Part model, mm, in its own coordinate system. A direction names the side the tool comes from. Coordinates: 2 decimals unless noted, no trailing zeros. Write each loop counter-clockwise with the first axis right and the second up, starting at its lowest first coordinate (ties: lowest second). Pieces come first, ordered by that corner, then holes. Notation, with made-up numbers: (11.25, 50) - (22.25, 50) arc R28 ccw to (22.25, 78) - close; hole circle Ø2 at (14, 16). An arc over 180 degrees is marked (long way). Write each question's results on one line, items separated by ' | '.
from build123d import *

# Parameters (mm, degrees)
SKETCH1_W                  = 260
SKETCH1_H                  = 200
EXTRUDE1_DEPTH             = 10
SKETCH2_R                  = 79.5
EXTRUDE2_DEPTH             = 10
M4_CLEARANCE_HOLE2_DEPTH   = 10
EXTRUDE3_DEPTH             = 10
SKETCH6_W                  = 30
SKETCH6_H                  = 77.5
EXTRUDE4_DEPTH             = 10
FILLET1_R                  = 8
M4_CLEARANCE_HOLE3_D       = 4.5
M4_CLEARANCE_HOLE3_DEPTH   = 20
EXTRUDE5_DEPTH             = 10
F_12_0_12_DIAMETER_HOLE1_D = 12
CHAMFER1_SIZE              = 30
CHAMFER2_SIZE              = 1
CHAMFER3_SIZE              = 60
SKETCH16_W                 = 146
SKETCH16_H                 = 3
EXTRUDE6_DEPTH             = 10
FILLET4_R                  = 10
EXTRUDE7_DEPTH             = 10
SKETCH18_W                 = 20
SKETCH18_H                 = 10
EXTRUDE8_DEPTH             = 10
EXTRUDE9_DEPTH             = 10


# Read off the part's stored shape, not the designer's step: M4 Clearance Hole2
with BuildPart() as part:
    # Sketch1 → Extrude1 (new body)
    with BuildSketch(Plane(origin=(0, 0, 0), x_dir=(1, 0, 0), z_dir=(0, 1, 0))):
        Rectangle(SKETCH1_W, SKETCH1_H)
    extrude(amount=EXTRUDE1_DEPTH)

    # Sketch2 → Extrude2 (cut)
    with BuildSketch(Plane(origin=(0, 10, 0), x_dir=(1, 0, 0), z_dir=(0, 1, 0))):
        with Locations(Location((0, 0, 0), (0, 0, 270))):
            Circle(SKETCH2_R)
    extrude(amount=-EXTRUDE2_DEPTH, mode=Mode.SUBTRACT)

    # M4 Clearance Hole2 outline → M4 Clearance Hole2 (cut)
    with BuildSketch(Plane(origin=(0, 0, 0), x_dir=(1, 0, 0), z_dir=(0, 1, 0))):
        with BuildLine():
            ThreePointArc((-82.75, 48.75), (-85, 51), (-87.25, 48.75))
            Line((-87.25, 48.75), (-87.25, 41.25))
            ThreePointArc((-87.25, 41.25), (-85, 39), (-82.75, 41.25))
            Line((-82.75, 41.25), (-82.75, 48.75))
        make_face()
        with BuildLine():
            ThreePointArc((87.25, 48.75), (85, 51), (82.75, 48.75))
            Line((82.75, 48.75), (82.75, 41.25))
            ThreePointArc((82.75, 41.25), (85, 39), (87.25, 41.25))
            Line((87.25, 41.25), (87.25, 48.75))
        make_face()
    extrude(amount=M4_CLEARANCE_HOLE2_DEPTH, mode=Mode.SUBTRACT)

    # Sketch5 → Extrude3 (cut)
    with BuildSketch(Plane.XZ):
        with BuildLine():
            Line((-130, 2.5), (105, 2.5))
            ThreePointArc((105, 2.5), (107.5, 0), (105, -2.5))
            Line((105, -2.5), (-130, -2.5))
            Line((-130, -2.5), (-130, 2.5))
        make_face()
    extrude(amount=-EXTRUDE3_DEPTH, mode=Mode.SUBTRACT)

    # Sketch6 → Extrude4 (cut)
    with BuildSketch(Plane.XZ):
        with Locations((-115, 61.25)):
            Rectangle(SKETCH6_W, SKETCH6_H)
    extrude(amount=-EXTRUDE4_DEPTH, mode=Mode.SUBTRACT)

    # Fillet1
    fillet1_edges = [part.edges().sort_by_distance(p)[0] for p in [
        (-100, 5, 22.5),
    ]]
    fillet(fillet1_edges, radius=FILLET1_R)

    # M4 Clearance Hole3
    with Locations(Plane.XY.offset(22.5)):
        with Locations((-123, 5)):
            Hole(M4_CLEARANCE_HOLE3_D / 2, depth=M4_CLEARANCE_HOLE3_DEPTH)

    # Sketch11 → Extrude5 (cut)
    with BuildSketch(Plane.XZ):
        Polygon((-125.25, -2.5), (-125.25, -9.5), (-126.625, -9.5), (-126.625, -13.2), (-125.25, -13.2), (-125.25, -18.5), (-120.75, -18.5), (-120.75, -13.2), (-119.375, -13.2), (-119.375, -9.5), (-120.75, -9.5), (-120.75, -2.5), align=None)
    extrude(amount=-EXTRUDE5_DEPTH, mode=Mode.SUBTRACT)

    # Ø12.0 (12) Diameter Hole1 (through all)
    with Locations(Plane(origin=(-130, 20, 100), x_dir=(1, 0, 0), z_dir=(0, 1, 0))):
        with Locations((65, 165), (195, 165), (195, 35), (65, 35)):
            Hole(F_12_0_12_DIAMETER_HOLE1_D / 2)

    # Chamfer1
    chamfer1_edges = [part.edges().sort_by_distance(p)[0] for p in [
        (-100, 5, 100),
    ]]
    chamfer(chamfer1_edges, length=CHAMFER1_SIZE)

    # Chamfer2
    chamfer2_edges = [part.edges().sort_by_distance(p)[0] for p in [
        (-130, 5, 2.5),
        (-130, 5, -2.5),
        (-130, 5, 22.5),
    ]]
    chamfer(chamfer2_edges, length=CHAMFER2_SIZE)

    # Chamfer3
    chamfer3_edges = [part.edges().sort_by_distance(p)[0] for p in [
        (130, 5, 100),
    ]]
    chamfer(chamfer3_edges, length=CHAMFER3_SIZE)

    # Sketch16 → Extrude6 (cut)
    with BuildSketch(Plane(origin=(0, 10, 0), x_dir=(1, 0, 0), z_dir=(0, 1, 0))):
        with Locations((0, -98.5)):
            Rectangle(SKETCH16_W, SKETCH16_H)
    extrude(amount=-EXTRUDE6_DEPTH, mode=Mode.SUBTRACT)

    # Fillet4
    fillet4_edges = [part.edges().sort_by_distance(p)[0] for p in [
        (-100, 5, 70),
        (130, 5, 40),
        (-73, 5, 97),
        (73, 5, 97),
    ]]
    fillet(fillet4_edges, radius=FILLET4_R)

    # Sketch17 → Extrude7 (cut)
    with BuildSketch(Plane(origin=(0, 10, 0), x_dir=(1, 0, 0), z_dir=(0, 1, 0))):
        Polygon((-122.5, -2.5), (-123.5, -2.5), (-123, -3.5), align=None)
    extrude7 = extrude(amount=-EXTRUDE7_DEPTH, mode=Mode.SUBTRACT)

    # Mirror1: Extrude7 across plane
    add(extrude7.mirror(Plane(origin=(0, 0, 12.5), x_dir=(1, 0, 0), z_dir=(0, 0, -1))), mode=Mode.SUBTRACT)

    # Sketch18 → Extrude8 (add)
    with BuildSketch(Plane(origin=(0, 10, 0), x_dir=(1, 0, 0), z_dir=(0, 1, 0))):
        with Locations((0, 105)):
            Rectangle(SKETCH18_W, SKETCH18_H)
    extrude(amount=-EXTRUDE8_DEPTH)

    # Sketch19 → Extrude9 (cut)
    with BuildSketch(Plane(origin=(0, 10, 0), x_dir=(1, 0, 0), z_dir=(0, 1, 0))):
        with BuildLine():
            Line((-11.5, 100), (-10, 100))
            Line((-10, 100), (-10, 101.5))
            ThreePointArc((-10, 101.5), (-8.939339828, 98.939339828), (-11.5, 100))
        make_face()
        with BuildLine():
            Line((10, 101.5), (10, 100))
            Line((10, 100), (11.5, 100))
            ThreePointArc((11.5, 100), (8.939339828, 98.939339828), (10, 101.5))
        make_face()
    extrude(amount=-EXTRUDE9_DEPTH, mode=Mode.SUBTRACT)


solid = part.part
(1) Saw through at B-B on z = 11.5. Write the cut outline in (x, y), then the cut area to 3 significant figures.
Return value:
outline: (-130, 0) - (-78.66, 0) - (-78.66, 10) - (-130, 10) - close; (78.66, 0) - (130, 0) - (130, 10) - (78.66, 10) - close; hole circle Ø4.5 at (-123, 5) | area: 1,010 mm^2
(2) Wall check: line 1 (X direction, y = 2.25, z = -65); line 2 (Y direction, x = -123, z = 13); line 3 (X direction, y = 6, z = 65). Give the ranges that are in metal, low to high. Write a range as from..to.
Return value:
line 1: x = -130..-71, -59..-45.77, 45.77..59, 71..130 | line 2: y = 0..2.75, 7.25..10 | line 3: x = -100..-71, -59..-45.77, 45.77..59, 71..105
(3) 3-axis set-ups, long thin cutter, end or side, ignore diameter. For faces 4 (the flat face through (-126, 5, 22.5)), 5 (the flat face through (92, 5, -2.5)), 6 (the flat face through (-10, 5, -106)): which of +Z, -Z, +X, -X, +Y, -Y reach the whole face in a straight line?
Return value:
face 4: +Z, -X, +Y, -Y | face 5: -X, +Y, -Y | face 6: -Z, -X, +Y, -Y
(4) Two-plate mould, pull along Z, no slides. Class faces 1 (the cylindrical face through (129.26, 5.07, 39.63)), 2 (the flat face through (10, 5, -106)), 3 (the flat face through (-87.25, 5, -45)): released by +Z, released by -Z, zero draft, split by the parting line, or undercut.
Return value:
face 1: released by +Z | face 2: zero draft | face 3: undercut
(5) Saw through at A-A on x = 0. Write the cut outline in (y, z).
Return value:
outline: (0, -110) - (10, -110) - (10, -79.5) - (0, -79.5) - close; (0, 79.5) - (10, 79.5) - (10, 97) - (0, 97) - close
(6) Flat gauge pins, fed straight in: P1, Ø4, axis at y = 5, z = -107, coming from the +X side; P2, Ø1.1, axis at x = -120, y = 7, coming from the -Z side; P3, Ø2, axis at x = -122, y = 6, coming from the +Z side. Where does each tip first touch, or does it go through?
Return value:
P1: stops at x = 10 | P2: stops at z = -100 | P3: stops at z = 22.5
(7) Saw through at D-D on x = -48.5. Write the cut outline in (y, z).
Return value:
outline: (0, -100) - (10, -100) - (10, -62.99) - (0, -62.99) - close; (0, 62.99) - (10, 62.99) - (10, 97) - (0, 97) - close
(8) Saw through at C-C on z = -65. Write the cut outline in (x, y), then the cut area to 3 significant figures.
Return value:
outline: (-130, 0) - (-71, 0) - (-71, 10) - (-130, 10) - close; (-59, 0) - (-45.77, 0) - (-45.77, 10) - (-59, 10) - close; (45.77, 0) - (59, 0) - (59, 10) - (45.77, 10) - close; (71, 0) - (130, 0) - (130, 10) - (71, 10) - close | area: 1,440 mm^2
